```python
from build123d import *

# Parameters (mm, degrees)
SKETCH17_W         = 12
SKETCH17_H         = 1.17
SKETCH1_R          = 2
EXTRUDE3_DEPTH     = 1.6
CUT_EXTRUDE1_DEPTH = 0.533333333
CIRPATTERN1_COUNT  = 6


with BuildPart() as part:
    # Sketch17 → Revolve1 (revolve)
    with BuildSketch(Plane(origin=(0, 0, 0), x_dir=(0, 0, -1), z_dir=(1, 0, 0))):
        with Locations((6, 0.585)):
            Rectangle(SKETCH17_W, SKETCH17_H)
    revolve(axis=Axis((0, 0, 0), (0, 0, 1)))

    # Sketch1 → Extrude3 (add)
    with BuildSketch(Plane.XY):
        Circle(SKETCH1_R)
    extrude(amount=EXTRUDE3_DEPTH)

    # Sketch11 → Cut-Revolve3 (revolve, cut)
    with BuildSketch(Plane(origin=(0, 0, 0), x_dir=(0, 0, -1), z_dir=(1, 0, 0))):
        with BuildLine():
            Line((-0.933333333, 2), (-0.32, 2))
            ThreePointArc((-0.32, 2), (-0.09372583, 1.90627417), (0, 1.68))
            Line((0, 1.68), (0.254, 1.68))
            Line((0.254, 1.68), (0.254, 2.254))
            Line((0.254, 2.254), (-1.854, 2.254))
            Line((-1.854, 2.254), (-1.854, 1.333333333))
            Line((-1.854, 1.333333333), (-1.6, 1.333333333))
            ThreePointArc((-1.6, 1.333333333), (-1.404737854, 1.804737854), (-0.933333333, 2))
        make_face()
    revolve(axis=Axis((0, 0, 0), (0, 0, 1)), mode=Mode.SUBTRACT)

    # Sketch12 → Cut-Extrude1 (cut)
    with BuildSketch(Plane.XY.offset(1.6)):
        with BuildLine():
            Line((-0.327453492, 0.567166085), (0, 0))
            Line((0, 0), (0.327453492, 0.567166085))
            ThreePointArc((0.327453492, 0.567166085), (0.229009756, 0.651587798), (0.167817831, 0.765928268))
            ThreePointArc((0.167817831, 0.765928268), (0, 0.888888889), (-0.167817831, 0.765928268))
            ThreePointArc((-0.167817831, 0.765928268), (-0.229009756, 0.651587798), (-0.327453492, 0.567166085))
        make_face()
    cut_extrude1 = extrude(amount=-CUT_EXTRUDE1_DEPTH, mode=Mode.SUBTRACT)

    # CirPattern1: Cut-Extrude1 ×6 about axis
    cirpattern1_axis = Axis((0, 0, 0), (0, 0, 1))
    for i in range(1, CIRPATTERN1_COUNT):
        add(cut_extrude1.rotate(cirpattern1_axis, i * 360 / CIRPATTERN1_COUNT), mode=Mode.SUBTRACT)


solid = part.part
```
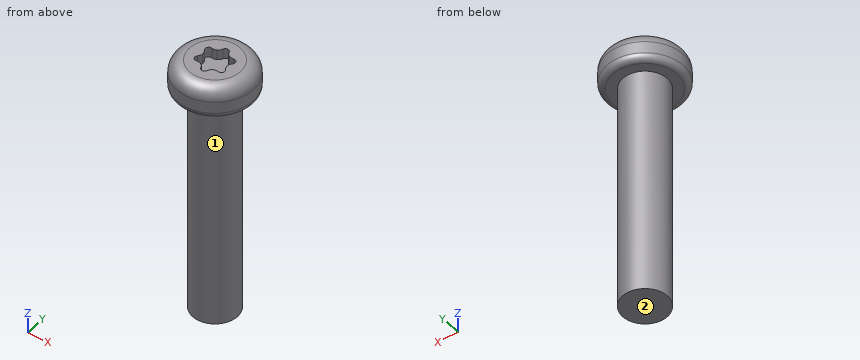
The model under review builds one solid part; all positions refer to its coordinate system, in mm. Face numbers are marked on the shaded views. A direction names the side the tool comes from. Give positions to 0.01 mm unless a question says otherwise; leave off trailing zeros. Order: outer loops, then holes, each group sorted by start corner. A loop starts at its lowest first (then second) coordinate and runs counter-clockwise, first axis right, second up. Notation, with made-up numbers: (-14, 10.25) - (28, 10.25) arc R10 ccw to (28, 15.25) - close; hole circle Ø3 at (-23.5, 16.5). An arc over 180 degrees is marked (long way). Use CSV: the item, a comma, the result in double quotes. Start each with the question number.
Q1. We need section A-A, the plane x = 0. Write out the cut boundary in (y, z).
Q2. Tool access review of the marked faces 1 and 2: name each direction out of +Z, -Z, +X, -X, +Y, -Y from which nothing blocks a thin tool from reaching the whole face with its end or side.
Q3. To check wall thickness, follow line 1 along Z through (x, y) = (1.35, -0.3); line 2 along X through (y, z) = (-0.05, -9); line 3 along Z through (x, y) = (-0.5, 0.25). State the ranges of each line that lie inside material, in increasing order. Write a range as [from, to].
Q4. Clearance check with flat-ended pins moving along their axes: pin 1 Ø1.5 at (y, z) = (1, -3) entering from +X; pin 2 Ø1 at (y, z) = (0.5, -2) entering from +X; pin 3 Ø2 at (x, z) = (1, -6.5) entering from +Y. State where each tip first meets the part, or that it passes through.
Q5. We need section B-B, the plane z = -9.75. Write out the cut boundary in (x, y).
Outcome:
1,outline,"(-2, 0.32) arc R0.32 ccw to (-1.68, 0) - (-1.17, 0) - (-1.17, -12) - (1.17, -12) - (1.17, 0) - (1.68, 0) arc R0.32 ccw to (2, 0.32) - (2, 0.93) arc R0.67 ccw to (1.33, 1.6) - (0.89, 1.6) - (0.89, 1.07) - (-0.89, 1.07) - (-0.89, 1.6) - (-1.33, 1.6) arc R0.67 ccw to (-2, 0.93) - close"
2,face 1,"-Z"
2,face 2,"-Z, +X, -X, +Y, -Y"
3,line 1,"z = [0, 1.6]"
3,line 2,"x = [-1.17, 1.17]"
3,line 3,"z = [-12, 1.07]"
4,pin 1,"stops at x = 1.14"
4,pin 2,"stops at x = 1.17"
4,pin 3,"stops at y = 1.17"
5,outline,"circle Ø2.34 at (0, 0)"
